Autodesk Inventor part; units mm, degrees
ref_plane "YZ Plane" through (0, 0, 0) normal (1, 0, 0) x (0, 1, 0)
ref_plane "XZ Plane" through (0, 0, 0) normal (0, 1, 0) x (-1, 0, 0)
ref_plane "XY Plane" through (0, 0, 0) normal (0, 0, 1) x (1, 0, 0)
sketch "Esquisse1" plane through (0, 0, 0) normal (0, 0, 1) x (1, 0, 0)
  line L0 (0, 0) -> (42, 0)
  line L1 (42, 0) -> (42, 42)
  line L2 (42, 42) -> (0, 42)
  line L3 (0, 42) -> (0, 0)
  dimension "d0" = 42
  dimension "d1" = 42
extrude "Extrusion1" add sketch "Esquisse1" along normal blind 48
sketch "Esquisse2" plane through (0, 0, 0) normal (0, 0, -1) x (-1, 0, 0)
  line L0 (0, 42) -> (0, 0)
  line L1 (0, 0) -> (-42, 0)
  circle A0 centre (-21, 21) radius 12.5
  dimension "d4" = 21
  dimension "d5" = 21
  dimension "d6" = 25
extrude "Extrusion2" cut sketch "Esquisse2" against normal blind 2
sketch "Esquisse5" plane through (21, 21, 2) normal (0, 0, -1) x (-1, 0, 0)
  circle A0 centre (0, 0) radius 12.5
  circle A1 centre (0, 0) radius 3.5
  point P0 (21, -21)
  dimension "d18" = 7
extrude "Extrusion5" cut sketch "Esquisse5" against normal blind 15 contours A1
sketch "Esquisse6" plane through (21, 21, 17) normal (0, 0, -1) x (-1, 0, 0)
  circle A0 centre (0, 0) radius 3.5
  circle A1 centre (0, 0) radius 2.5
  point P0 (21, -21)
  dimension "d21" = 5
extrude "Extrusion6" add sketch "Esquisse6" along normal blind 41 contours A1
sketch "Esquisse7" plane through (42, 0, 0) normal (1, 0, 0) x (0, 0, -1)
  line L0 (0, 0) -> (-48, 0)
  line L1 (-48, 0) -> (-48, 42)
  circle A0 centre (-33, 21) radius 2.5
  line L2 (-15.5634, 24.7779) -> (-36.4192, 24.7779) construction
  line L3 (-36.4192, 24.7779) -> (-36.4192, 35.8396) construction
  line L4 (-36.4192, 35.8396) -> (-15.5634, 35.8396) construction
  line L5 (-15.5634, 35.8396) -> (-15.5634, 24.7779) construction
  dimension "d24" = 21
  dimension "d25" = 15
  dimension "d26" = 5
extrude "Extrusion7" cut sketch "Esquisse7" against normal blind 20
sketch "Esquisse8" plane through (42, 0, 0) normal (1, 0, 0) x (0, 0, -1)
  line L0 (-18.5513, 11.8106) -> (-48.2794, 11.8106) construction
  line L1 (-48.2794, 11.8106) -> (-48.2794, 27.9421) construction
  line L2 (-48.2794, 27.9421) -> (-18.5513, 27.9421) construction
  line L3 (-18.5513, 27.9421) -> (-18.5513, 11.8106) construction
  point P0 (0, 0)
properties part number "moteur 17HS19-2004S1"
Work out the finished part from the listing and answer in its coordinate system (mm). A direction names the side the tool comes from. Give positions to 0.01 mm unless a question says otherwise; leave off trailing zeros. Loops run counter-clockwise (first coordinate to the right, second up) from the corner with the lowest first, then second, coordinate; pieces in that order, holes last. Notation, with made-up numbers: (58.25, 17.25) -> (114.25, 17.25) arc R10 cw to (114.25, 30.25) -> close; hole circle Ø8 at (35, 53.5). An arc over 180 degrees is marked (long way). One line per question, with ' | ' between items. Start each with the question number.
1) For faces 1 (the face through (21, 0, 24)), 2 (the face through (22, 21, 33)), 3 (the face through (23.5, 20.9, -3.2)), determine the directions among +Z, -Z, +X, -X, +Y, -Y from which every point of the face is accessible in a straight line to the end or side of a thin tool.
2) Section B-B, the plane z = 33 is taken. Determine the outline of the cut face in (x, y).
3) Section D-D, the plane x = 38 is taken. Determine the outline of the cut face in (y, z).
4) Determine the mould class of faces 4 (the face through (32.14, 23.48, 33.33)), 5 (the face through (19, 19, 17)), 6 (the face through (21, 21, 48)), 7 (the face through (19.12, 23.95, 9.4)) for opening direction Z: +Z half, -Z half, draft (parallel to the pull), parting line (faces both ways), or undercut.
5) Each of these flat-tipped pins is pushed along its axis until it touches: pin 1 (3 mm diameter, centred on y = 20, z = -14.5, fed in from -X); pin 2 (10 mm diameter, centred on x = 16.5, y = 12, fed in from -Z); pin 3 (4 mm diameter, centred on y = 21, z = 33, fed in from +X). Where does it stop, or does it pass through?
6) Straight lines are drawn through the part: L1, parallel to Y at x = 21, z = 6; L2, parallel to Y at x = 21, z = 1.2; L3, parallel to Y at x = 37.5, z = 33. For each, find the intervals that lie inside material, in ascending order.
7) Section C-C, the plane x = 21 is taken. Determine the outline of the cut face in (y, z).
8) Section A-A, the plane y = 11 is taken. Determine the outline of the cut face in (x, z), then the cut area to 3 significant figures.
Resolved:
1) face 1: +Z, -Z, +X, -X, -Y | face 2: +X | face 3: -Z
2) outline: (0, 0) -> (42, 0) -> (42, 18.5) -> (22, 18.5) -> (22, 23.5) -> (42, 23.5) -> (42, 42) -> (0, 42) -> close
3) outline: (0, 0) -> (42, 0) -> (42, 48) -> (0, 48) -> close; hole circle Ø5 at (21, 33)
4) face 4: undercut | face 5: -Z half | face 6: +Z half | face 7: draft
5) pin 1: x = 18.5 | pin 2: z = 0 | pin 3: x = 22
6) L1: 0 to 17.5, 18.5 to 23.5, 24.5 to 42 | L2: 0 to 8.5, 18.5 to 23.5, 33.5 to 42 | L3: 0 to 18.5, 23.5 to 42
7) outline: (0, 0) -> (8.5, 0) -> (8.5, 2) -> (17.5, 2) -> (17.5, 17) -> (18.5, 17) -> (18.5, -24) -> (23.5, -24) -> (23.5, 17) -> (24.5, 17) -> (24.5, 2) -> (33.5, 2) -> (33.5, 0) -> (42, 0) -> (42, 48) -> (0, 48) -> close
8) outline: (0, 0) -> (13.5, 0) -> (13.5, 2) -> (28.5, 2) -> (28.5, 0) -> (42, 0) -> (42, 48) -> (0, 48) -> close | area: 1,990 mm2
